For this review, take the finished solid that the model builds, in its own axes (mm). Coordinates: 2 decimals unless noted, no trailing zeros. Answer as a JSON object with one key per item and string values. Group by question number.
Item 1: We need section A-A (z = 2.75). State how many separate pieces and enclosed holes the cut face has, then the cut area to 3 significant figures.
Item 2: Clearance check with flat-ended pins moving along their axes: pin 1 (2 mm diameter, centred on y = -1, z = 1.5, fed in from +X); pin 2 (1 mm diameter, centred on x = 1.5, z = 5.5, fed in from +Y). State where each tip first meets the part, or that it passes through.
Item 3: To check wall thickness, follow line 1 (Y direction, x = 1.65, z = 6.25); line 2 (Y direction, x = 0.9, z = 5); line 3 (Y direction, x = 0.1, z = 1). State the ranges of each line that lie inside material, in increasing order.
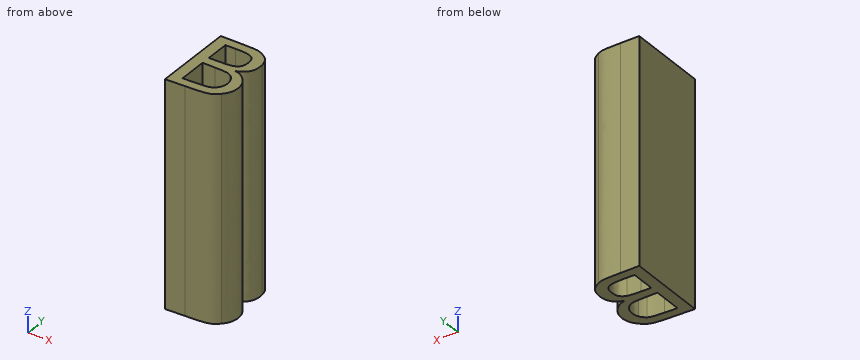
from build123d import *

# Parameters (mm, degrees)
PAD001_DEPTH    = 10
POCKET_DEPTH    = 10.001
POCKET001_DEPTH = 10.001


with BuildPart() as part:
    # Sketch009 → Pad001 (new body)
    with BuildSketch(Plane.XY):
        with BuildLine():
            add(Edge.make_bspline(
                [(0, -1.849196), (0, -0.034171)],
                knots=[0, 0, 6.43119, 6.43119], degree=1))
            add(Edge.make_bspline(
                [(0, -0.034171), (0.841544, -0.048254)],
                knots=[0, 0, 2.982267, 2.982267], degree=1))
            add(Edge.make_bspline(
                [(0.841544, -0.048254), (1.669189, -0.062111), (1.687071, -0.064285), (1.924166, -0.180713)],
                knots=[0, 0, 0, 0, 1, 1, 1, 1], degree=3))
            add(Edge.make_bspline(
                [(1.924166, -0.180713), (2.2246, -0.328239), (2.3645, -0.523607), (2.397303, -0.84144)],
                knots=[0, 0, 0, 0, 1, 1, 1, 1], degree=3))
            add(Edge.make_bspline(
                [(2.397303, -0.84144), (2.438256, -1.238239), (2.295169, -1.519628), (1.979351, -1.663384)],
                knots=[0, 0, 0, 0, 1, 1, 1, 1], degree=3))
            add(Edge.make_bspline(
                [(1.979351, -1.663384), (1.818476, -1.736609)],
                knots=[0, 0, 0.626302, 0.626302], degree=1))
            add(Edge.make_bspline(
                [(1.818476, -1.736609), (1.952851, -1.766124)],
                knots=[0, 0, 0.48748, 0.48748], degree=1))
            add(Edge.make_bspline(
                [(1.952851, -1.766124), (2.026759, -1.782352), (2.162852, -1.863818), (2.255283, -1.947153)],
                knots=[0, 0, 0, 0, 1, 1, 1, 1], degree=3))
            add(Edge.make_bspline(
                [(2.255283, -1.947153), (2.675938, -2.326397), (2.692169, -2.936934), (2.291915, -3.324947)],
                knots=[0, 0, 0, 0, 1, 1, 1, 1], degree=3))
            add(Edge.make_bspline(
                [(2.291915, -3.324947), (2.007164, -3.600986), (1.898949, -3.625672), (0.883102, -3.646294)],
                knots=[0, 0, 0, 0, 1, 1, 1, 1], degree=3))
            add(Edge.make_bspline(
                [(0.883102, -3.646294), (0, -3.664215)],
                knots=[0, 0, 3.129744, 3.129744], degree=1))
            add(Edge.make_bspline(
                [(0, -3.664215), (0, -1.849196)],
                knots=[0, 0, 6.43117, 6.43117], degree=1))
        make_face()
    extrude(amount=PAD001_DEPTH)

    # Sketch010 (on Face14 of Pad001) → Pocket (cut, through all)
    with BuildSketch(Plane.XY.offset(10)):
        with BuildLine():
            add(Edge.make_bspline(
                [(1.786983, -3.136194), (1.866979, -3.089704), (1.965133, -2.986848), (2.005096, -2.907625)],
                knots=[0, 0, 0, 0, 1, 1, 1, 1], degree=3))
            add(Edge.make_bspline(
                [(2.005096, -2.907625), (2.157451, -2.605611), (2.057265, -2.215594), (1.786983, -2.05852)],
                knots=[0, 0, 0, 0, 1, 1, 1, 1], degree=3))
            add(Edge.make_bspline(
                [(1.786983, -2.05852), (1.664183, -1.987158), (1.55253, -1.971754), (1.070113, -1.959618)],
                knots=[0, 0, 0, 0, 1, 1, 1, 1], degree=3))
            add(Edge.make_bspline(
                [(1.070113, -1.959618), (0.498692, -1.945253)],
                knots=[0, 0, 2.02536, 2.02536], degree=1))
            add(Edge.make_bspline(
                [(0.498692, -1.945253), (0.498692, -2.597367)],
                knots=[0, 0, 2.31064, 2.31064], degree=1))
            add(Edge.make_bspline(
                [(0.498692, -2.597367), (0.498692, -3.249484)],
                knots=[0, 0, 2.31065, 2.31065], degree=1))
            add(Edge.make_bspline(
                [(0.498692, -3.249484), (1.070113, -3.235119)],
                knots=[0, 0, 2.02536, 2.02536], degree=1))
            add(Edge.make_bspline(
                [(1.070113, -3.235119), (1.55253, -3.222983), (1.664183, -3.207574), (1.786983, -3.136214)],
                knots=[0, 0, 0, 0, 1, 1, 1, 1], degree=3))
            add(Edge.make_bspline(
                [(1.786983, -3.136214), (1.786983, -3.136194)],
                knots=[0, 0, 7e-05, 7e-05], degree=1))
        make_face()
    extrude(amount=-POCKET_DEPTH, mode=Mode.SUBTRACT)

    # Sketch007 (on Face14 of Pad001) → Pocket001 (cut, through all)
    with BuildSketch(Plane.XY.offset(10)):
        with BuildLine():
            add(Edge.make_bspline(
                [(1.540722, -1.49591), (1.788411, -1.427102), (1.890878, -1.281218), (1.890878, -0.997385)],
                knots=[0, 0, 0, 0, 1, 1, 1, 1], degree=3))
            add(Edge.make_bspline(
                [(1.890878, -0.997385), (1.890878, -0.567038), (1.699553, -0.457759), (0.945439, -0.457367)],
                knots=[0, 0, 0, 0, 1, 1, 1, 1], degree=3))
            add(Edge.make_bspline(
                [(0.945439, -0.457367), (0.498692, -0.457135)],
                knots=[0, 0, 1.58296, 1.58296], degree=1))
            add(Edge.make_bspline(
                [(0.498692, -0.457135), (0.498692, -0.997387)],
                knots=[0, 0, 1.91428, 1.91428], degree=1))
            add(Edge.make_bspline(
                [(0.498692, -0.997387), (0.498692, -1.537637)],
                knots=[0, 0, 1.91427, 1.91427], degree=1))
            add(Edge.make_bspline(
                [(0.498692, -1.537637), (0.945439, -1.537389)],
                knots=[0, 0, 1.58296, 1.58296], degree=1))
            add(Edge.make_bspline(
                [(0.945439, -1.537389), (1.19115, -1.537262), (1.459024, -1.518593), (1.540722, -1.495893)],
                knots=[0, 0, 0, 0, 1, 1, 1, 1], degree=3))
            add(Edge.make_bspline(
                [(1.540722, -1.495893), (1.540722, -1.49591)],
                knots=[0, 0, 6e-05, 6e-05], degree=1))
        make_face()
    extrude(amount=-POCKET001_DEPTH, mode=Mode.SUBTRACT)


solid = part.part
Check sheet entries:
{
 "1": {"separate pieces": "1", "enclosed holes": "2", "area": "5.06 mm2"},
 "2": {"pin 1": "stops at x = 2.4", "pin 2": "stops at y = -0.05"},
 "3": {"line 1": "y = -3.61 to -3.19, -2 to -1.46, -0.54 to -0.08", "line 2": "y = -3.65 to -3.24, -1.96 to -1.54, -0.46 to -0.05", "line 3": "y = -3.66 to -0.04"}
}
